from build123d import *

# Parameters (mm, degrees)
AUFSATZ_LINEAR_AUSTRAGEN1_DEPTH      = 35
AUFSATZ_LINEAR_AUSTRAGEN1_DEPTH_BACK = 35
SKIZZE1_R                            = 25
SKIZZE2_W                            = 66
SKIZZE2_H                            = 50
AUFSATZ_LINEAR_AUSTRAGEN2_DEPTH      = 700
AUFSATZ_LINEAR_AUSTRAGEN3_DEPTH      = 10
SCHNITT_LINEAR_AUSTRAGEN1_REACH      = 776.344
SKIZZE4_R                            = 6
VERRUNDUNG2_START                    = -1e-07
VERRUNDUNG2_DEPTH                    = 660.0000001
VERRUNDUNG2_START_2                  = -33
VERRUNDUNG2_2_DEPTH                  = 66
FASE1_SIZE                           = 20
SKIZZE5_R                            = 20
AUFSATZ_LINEAR_AUSTRAGEN4_DEPTH      = 40


with BuildPart() as part:
    # Skizze1 → Aufsatz-Linear austragen1 (new, two sides: drawn at the far end of the back side and taken through both)
    with BuildSketch(Plane.XY.offset(-AUFSATZ_LINEAR_AUSTRAGEN1_DEPTH_BACK)):
        Circle(SKIZZE1_R)
    extrude(amount=AUFSATZ_LINEAR_AUSTRAGEN1_DEPTH + AUFSATZ_LINEAR_AUSTRAGEN1_DEPTH_BACK)

    # Skizze2 → Aufsatz-Linear austragen2 (add)
    with BuildSketch(Plane(origin=(0, 0, 0), x_dir=(0, 0, -1), z_dir=(1, 0, 0))):
        Rectangle(SKIZZE2_W, SKIZZE2_H)
    extrude(amount=AUFSATZ_LINEAR_AUSTRAGEN2_DEPTH)

    # Skizze3 → Aufsatz-Linear austragen3 (add)
    with BuildSketch(Plane(origin=(0, 0, -33), x_dir=(-1, 0, 0), z_dir=(0, 0, -1))):
        with BuildLine():
            Line((-700, 25), (-660, 25))
            ThreePointArc((-660, 25), (-635, 0), (-660, -25))
            Line((-660, -25), (-700, -25))
            Line((-700, -25), (-745, -25))
            ThreePointArc((-745, -25), (-770, 0), (-745, 25))
            Line((-745, 25), (-700, 25))
        make_face()
    aufsatz_linear_austragen3 = extrude(amount=AUFSATZ_LINEAR_AUSTRAGEN3_DEPTH)

    # Skizze4 → Schnitt-Linear austragen1 (cut, up to next)
    with BuildSketch(Plane(origin=(0, 0, -43), x_dir=(-1, 0, 0), z_dir=(0, 0, -1)), mode=Mode.PRIVATE) as schnitt_linear_austragen1_sk1:
        with Locations((-745, 0)):
            Circle(SKIZZE4_R)
    schnitt_linear_austragen1_tool1 = extrude(schnitt_linear_austragen1_sk1.sketch, amount=-SCHNITT_LINEAR_AUSTRAGEN1_REACH, mode=Mode.PRIVATE) & part.part
    schnitt_linear_austragen1 = schnitt_linear_austragen1_tool1.solids().sort_by_distance((745, 0, -43))[0]
    add(schnitt_linear_austragen1, mode=Mode.SUBTRACT)

    # Spiegeln1: Aufsatz-Linear austragen3, Schnitt-Linear austragen1 across plane
    add(aufsatz_linear_austragen3.mirror(Plane.XY))
    add(schnitt_linear_austragen1.mirror(Plane.XY), mode=Mode.SUBTRACT)

    # Verrundung2: read off the stored shape, not the designer's step
    # Verrundung2 outline → Verrundung2 (cut)
    with BuildSketch(Plane.YZ.offset(VERRUNDUNG2_START)):
        with BuildLine():
            Line((-25, -33), (-18, -33))
            ThreePointArc((-18, -33), (-22.949747468, -30.949747468), (-25, -26))
            Line((-25, -26), (-25, -33))
        make_face()
        with BuildLine():
            ThreePointArc((25, -26), (22.949747468, -30.949747468), (18, -33))
            Line((18, -33), (25, -33))
            Line((25, -33), (25, -26))
        make_face()
        with BuildLine():
            Line((-25, 33), (-25, 26))
            ThreePointArc((-25, 26), (-22.949747468, 30.949747468), (-18, 33))
            Line((-18, 33), (-25, 33))
        make_face()
        with BuildLine():
            ThreePointArc((18, 33), (22.949747468, 30.949747468), (25, 26))
            Line((25, 26), (25, 33))
            Line((25, 33), (18, 33))
        make_face()
    extrude(amount=VERRUNDUNG2_DEPTH, mode=Mode.SUBTRACT)

    # Verrundung2 2 outline → Verrundung2 2 (add)
    with BuildSketch(Plane.XY.offset(VERRUNDUNG2_START_2)):
        with BuildLine():
            Line((17.349351573, -18), (-1e-07, -18))
            Line((-1e-07, -18), (0, -25))
            ThreePointArc((0, -25), (9.354143467, -23.184046239), (17.349351573, -18))
        make_face()
        with BuildLine():
            Line((660, -18), (642.650648427, -18))
            ThreePointArc((642.650648427, -18), (650.645856533, -23.184046239), (660, -25))
            Line((660, -25), (660, -18))
        make_face()
        with BuildLine():
            Line((660, 18), (660, 25))
            ThreePointArc((660, 25), (650.645856533, 23.184046239), (642.650648427, 18))
            Line((642.650648427, 18), (660, 18))
        make_face()
        with BuildLine():
            ThreePointArc((17.349351573, 18), (9.354143467, 23.184046239), (0, 25))
            Line((0, 25), (-1e-07, 18))
            Line((-1e-07, 18), (17.349351573, 18))
        make_face()
    extrude(amount=VERRUNDUNG2_2_DEPTH)

    # Fase1
    fase1_edges = [part.edges().sort_by_distance(p)[0] for p in [
        (700, -25, 0),
        (700, 25, 0),
    ]]
    chamfer(fase1_edges, length=FASE1_SIZE)

    # Skizze5 → Aufsatz-Linear austragen4 (add)
    with BuildSketch(Plane.XY.offset(43)):
        with Locations(Location((745, 0, 0), (0, 0, 180))):
            Circle(SKIZZE5_R)
    extrude(amount=AUFSATZ_LINEAR_AUSTRAGEN4_DEPTH)


solid = part.part
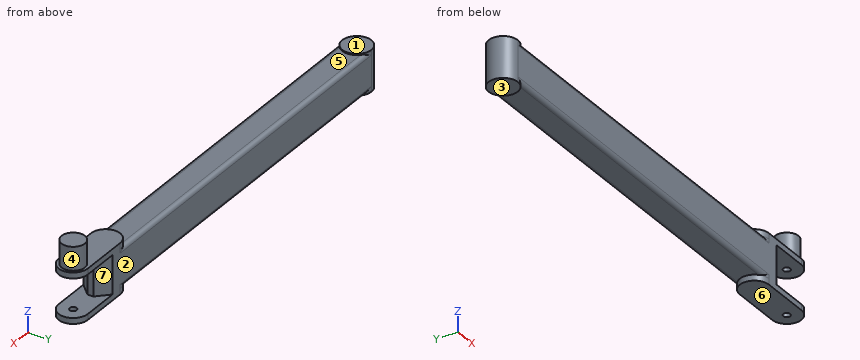
Can you work these out from the model? Positions are in its coordinate system, mm. Face numbers are marked on the shaded views. A direction names the side the tool comes from. Coordinates: 2 decimals unless noted, no trailing zeros. Loops run counter-clockwise (first coordinate to the right, second up) from the corner with the lowest first, then second, coordinate; pieces in that order, holes last. Notation, with made-up numbers: (-30, 49.25) - (6, 49.25) arc R18 ccw to (6, 53.25) - close; hole circle Ø2 at (60, 2). An arc over 180 degrees is marked (long way). Answer as a JSON object with one key per item and string values. Group by question number.
Item 1: If I drill on L1, parallel to Y at x = 745, z = 37; L2, parallel to Z at x = 720.5, y = -7.5; L3, parallel to Z at x = 255, y = 0.5, over which ranges is the centre line in solid material (lowest first)? Write a range as from..to.
Item 2: If we section it at B-B (z = -5.5): List the corners of the cut face in (x, y) for me, plus the area to 3 significant figures.
Item 3: For pin 1 (15.5 mm diameter, centred on x = 745, y = 0, fed in from -Z); pin 2 (12 mm diameter, centred on y = 19.5, z = 64, fed in from -X); pin 3 (5 mm diameter, centred on x = 357, z = 33, fed in from -Y); pin 4 (15 mm diameter, centred on x = -3, y = 12, fed in from +Z), each with a flat end and sliding along its axis, tell me the tip position at first contact or that it passes through.
Item 4: If we section it at A-A (x = 33): List the corners of the cut face in (y, z) for me.
Item 5: If we mould it in two halves opening along X, with no side actions, what happens to the marked faces 4, 5, 6 and 7? For each: released by +X, released by -X, zero draft, split by the parting line, or undercut.
Item 6: On a 3-axis mill with a long thin cutter (end or side, diameter ignored), from which of +Z, -Z, +X, -X, +Y, -Y can I reach the whole of each face in a straight line? I mean the marked faces 1, 2 and 3. Say none if no direction works.
Returned:
{
 "1": {"L1": "y = -25..-6, 6..25", "L2": "z = -43..-33, 33..43", "L3": "z = -33..33"},
 "2": {"outline": "(0, -25) - (680, -25) - (700, -5) - (700, 5) - (680, 25) - (0, 25) arc R25 ccw to start", "area": "35,600 mm²"},
 "3": {"pin 1": "stops at z = -43", "pin 2": "stops at x = 730.24", "pin 3": "stops at y = -23.36", "pin 4": "stops at z = 35"},
 "4": {"outline": "(-25, -26) arc R7 ccw to (-18, -33) - (18, -33) arc R7 ccw to (25, -26) - (25, 26) arc R7 ccw to (18, 33) - (-18, 33) arc R7 ccw to (-25, 26) - close"},
 "5": {"face 4": "split by the parting line", "face 5": "undercut", "face 6": "zero draft", "face 7": "released by +X"},
 "6": {"face 1": "+Z, -X, +Y, -Y", "face 2": "+Z, -Z, +X, -X, +Y", "face 3": "-Z, -X, +Y, -Y"}
}
